Source: CAD feature listing. Evaluate the final solid. Frame: model axes, mm. Face numbers are marked on the shaded views. A direction names the side the tool comes from. Round coordinates to 2 decimals unless told otherwise and drop trailing zeros. Order: outer loops, then holes, each group sorted by start corner. A loop starts at its lowest first (then second) coordinate and runs counter-clockwise, first axis right, second up. Notation, with made-up numbers: M 29.5,30.5 L 52.5,30.5 A31 ccw 52.5,60.5 Z; hole C -18,22 d4. An arc over 180 degrees is marked long. Use one line per item in the form item = value. Start each with the question number.
Q1. Contact query for flat-ended pins moving along their axis: pin 1 (1.1 mm diameter, centred on x = -2, y = 1, fed in from +Z); pin 2 (1 mm diameter, centred on x = -1, z = 6.5, fed in from -Y); pin 3 (0.8 mm diameter, centred on x = 2, y = 0.5, fed in from +Z). Output: stop coordinate, or through.
Q2. Section A-A (y = -0.7). Return the cut outline in (x, z).
Q3. Reachability of the marked faces 1, 2 and 3 from +Z, -Z, +X, -X, +Y, -Y: full face, straight path, thin tool, end or side. Return the list, or none.
Q4. Section C-C (y = 0). Return the cut outline in (x, z), plus the area to 3 significant figures.
Q5. Section D-D (x = 1.9). Return the cut outline in (y, z), plus the area to 3 significant figures.
Q6. Section B-B (z = 1.5). Return the cut outline in (x, y), plus the area to 3 significant figures.
Q7. Material intervals for probe 1 along X at (y, z) = (0.8, 4.5); probe 2 along Y at (x, z) = (0.1, 8.25); probe 3 along Y at (x, z) = (-0.6, 4.75), sorted ascending.
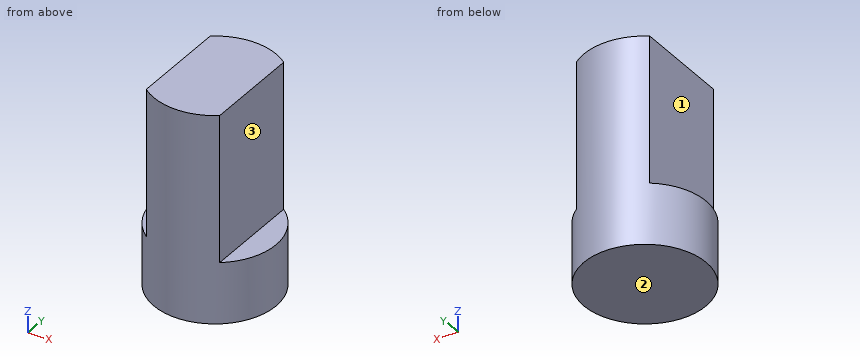
from build123d import *

# Parameters (mm, degrees)
SKETCH1_R           = 2.5
BOSS_EXTRUDE1_DEPTH = 8.5
CUT_EXTRUDE1_START  = -6
CUT_EXTRUDE1_DEPTH  = 6


with BuildPart() as part:
    # Sketch1 → Boss-Extrude1 (new body)
    with BuildSketch(Plane.XY):
        Circle(SKETCH1_R)
    extrude(amount=BOSS_EXTRUDE1_DEPTH)

    # Sketch2 → Cut-Extrude1 (cut)
    with BuildSketch(Plane.XY.offset(8.5).offset(CUT_EXTRUDE1_START)):
        with BuildLine():
            Line((-1.5, 2), (-1.5, -2))
            ThreePointArc((-1.5, -2), (-2.5, 0), (-1.5, 2))
        make_face()
        with BuildLine():
            Line((1.5, 2), (1.5, -2))
            ThreePointArc((1.5, -2), (2.5, 0), (1.5, 2))
        make_face()
    extrude(amount=CUT_EXTRUDE1_DEPTH, mode=Mode.SUBTRACT)


solid = part.part
Results list:
q1.pin_1 = 8.5
q1.pin_2 = -2.45
q1.pin_3 = 2.5
q2.outline = M -2.4,0 L 2.4,0 L 2.4,2.5 L 1.5,2.5 L 1.5,8.5 L -1.5,8.5 L -1.5,2.5 L -2.4,2.5 Z
q3.face_1 = +Z, -X, +Y, -Y
q3.face_2 = -Z, +X, -X, +Y, -Y
q3.face_3 = +Z, +X, +Y, -Y
q4.outline = M -2.5,0 L 2.5,0 L 2.5,2.5 L 1.5,2.5 L 1.5,8.5 L -1.5,8.5 L -1.5,2.5 L -2.5,2.5 Z
q4.area = 30.5 mm2
q5.outline = M -1.62,0 L 1.62,0 L 1.62,2.5 L -1.62,2.5 Z
q5.area = 8.12 mm2
q6.outline = C 0,0 d5
q6.area = 19.6 mm2
q7.probe_1 = -1.5 to 1.5
q7.probe_2 = -2.5 to 2.5
q7.probe_3 = -2.43 to 2.43
